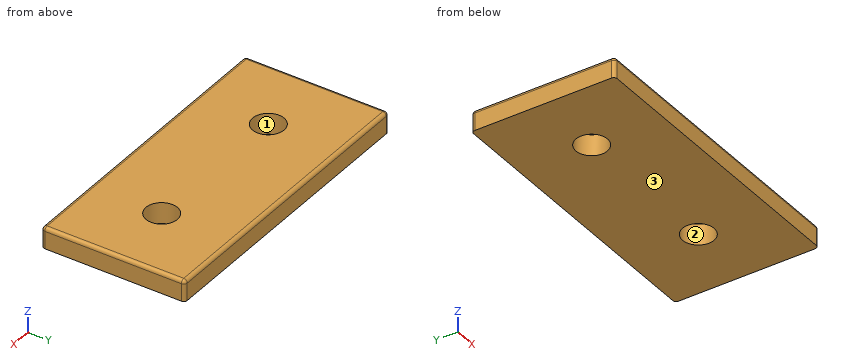
```python
from build123d import *

# Parameters (mm, degrees)
SKETCH1_W           = 86
SKETCH1_H           = 41
SKETCH1_R           = 4.5
BOSS_EXTRUDE1_DEPTH = 3
FILLET1_R           = 1


with BuildPart() as part:
    # Sketch1 → Boss-Extrude1 (new body, symmetric)
    with BuildSketch(Plane.XY):
        with Locations((43, 20.5)):
            Rectangle(SKETCH1_W, SKETCH1_H)
        with Locations((20.5, 20.5)):
            Circle(SKETCH1_R, mode=Mode.SUBTRACT)
        with Locations((65.5, 20.5)):
            Circle(SKETCH1_R, mode=Mode.SUBTRACT)
    extrude(amount=BOSS_EXTRUDE1_DEPTH, both=True)

    # Fillet1
    fillet1_edges = [part.edges().sort_by_distance(p)[0] for p in [
        (43, 41, 3),
        (0, 20.5, 3),
        (43, 0, 3),
        (86, 20.5, 3),
        (0, 0, 0),
        (0, 41, 0),
        (86, 41, 0),
        (86, 0, 0),
    ]]
    fillet(fillet1_edges, radius=FILLET1_R)


solid = part.part
```
Design review of the part built by this model. Coordinates are the model's own, in mm. Face numbers are marked on the shaded views. Coordinates: 2 decimals unless noted, no trailing zeros. Write each loop counter-clockwise with the first axis right and the second up, starting at its lowest first coordinate (ties: lowest second). Pieces come first, ordered by that corner, then holes.
1) To check wall thickness, follow L1, parallel to Y at x = 20.5, z = 0.2; L2, parallel to X at y = 27, z = 2.05. State the ranges of each line that lie inside material, in increasing order.
2) Add section A-A (y = 20.5). Write out the cut boundary in (x, z).
3) Insertion check: pin 1 (4 mm diameter, centred on x = 17.5, y = 21.5, fed in from -Z). The pin has a flat end and moves straight along its axis. Give the tip position at first contact, or say it passes through.
4) Add section B-B (x = 65.5). Write out the cut boundary in (y, z).
5) Mouldability with a two-part tool opening along Y and no side actions: class the marked faces 1, 2 and 3 as +Y half, -Y half, draft (parallel to the pull), parting line (faces both ways), or undercut.
6) Add section C-C (z = 0.15). Write out the cut boundary in (x, y), plus the area to 3 significant figures.
Check result:
1. L1: y = 0 to 16, 25 to 41
1. L2: x = 0 to 86
2. outline: (0, -3) - (16, -3) - (16, 3) - (1, 3) arc R1 ccw to (0, 2) - close; (25, -3) - (61, -3) - (61, 3) - (25, 3) - close; (70, -3) - (86, -3) - (86, 2) arc R1 ccw to (85, 3) - (70, 3) - close
3. pin 1: stops at z = -3
4. outline: (0, -3) - (16, -3) - (16, 3) - (1, 3) arc R1 ccw to (0, 2) - close; (25, -3) - (41, -3) - (41, 2) arc R1 ccw to (40, 3) - (25, 3) - close
5. face 1: undercut
5. face 2: undercut
5. face 3: draft
6. outline: (0, 1) arc R1 ccw to (1, 0) - (85, 0) arc R1 ccw to (86, 1) - (86, 40) arc R1 ccw to (85, 41) - (1, 41) arc R1 ccw to (0, 40) - close; hole circle Ø9 at (20.5, 20.5); hole circle Ø9 at (65.5, 20.5)
6. area: 3,400 mm2
